from build123d import *

# Parameters (mm, degrees)
SKETCH_R      = 49.5
SKETCH_R_2    = 47
PAD_DEPTH     = 100
SKETCH002_W   = 120
SKETCH002_H   = 120
SKETCH002_R   = 57.5
SKETCH002_R_2 = 2.5
PAD001_DEPTH  = 2.5
FILLET_R      = 4


with BuildPart() as part:
    # Sketch → Pad (new body)
    with BuildSketch(Plane.XY):
        Circle(SKETCH_R)
        Circle(SKETCH_R_2, mode=Mode.SUBTRACT)
    extrude(amount=PAD_DEPTH)

    # Sketch001 → Revolution (revolve)
    with BuildSketch(Plane.XZ):
        with BuildLine():
            ThreePointArc((-57.5, -10.5), (-50.075379, -7.424621), (-47, 0))
            Line((-49.5, 0), (-47, 0))
            ThreePointArc((-57.5, -8), (-51.843146, -5.656854), (-49.5, 0))
            Line((-57.5, -10.5), (-57.5, -8))
        make_face()
    revolve(axis=Axis((0, 0, 0), (0, 0, 1)))

    # Sketch002 (on DatumPlane) → Pad001 (join)
    with BuildSketch(Plane(origin=(0, 0, -10.5), x_dir=(0, -1, 0), z_dir=(0, 0, 1))):
        Rectangle(SKETCH002_W, SKETCH002_H)
        Circle(SKETCH002_R, mode=Mode.SUBTRACT)
        with Locations((-52.499987, 52.500013)):
            Circle(SKETCH002_R_2, mode=Mode.SUBTRACT)
        with Locations((-52.500013, -52.499987)):
            Circle(SKETCH002_R_2, mode=Mode.SUBTRACT)
        with Locations((52.499987, -52.500013)):
            Circle(SKETCH002_R_2, mode=Mode.SUBTRACT)
        with Locations((52.500013, 52.499987)):
            Circle(SKETCH002_R_2, mode=Mode.SUBTRACT)
    extrude(amount=PAD001_DEPTH)

    # Fillet
    fillet_edges = [part.edges().sort_by_distance(p)[0] for p in [
        (-60, -60, -9.25),
        (60, -60, -9.25),
        (-60, 60, -9.25),
        (60, 60, -9.25),
    ]]
    fillet(fillet_edges, radius=FILLET_R)


solid = part.part
Design review of the part built by this model. Coordinates are the model's own, in mm. A direction names the side the tool comes from. Coordinates: 2 decimals unless noted, no trailing zeros. Order: outer loops, then holes, each group sorted by start corner. A loop starts at its lowest first (then second) coordinate and runs counter-clockwise, first axis right, second up.
Item 1: For pin 1 Ø12 at (x, z) = (-25.5, 68) entering from +Y; pin 2 Ø4.5 at (x, y) = (-52.5, -52.5) entering from -Z; pin 3 Ø2 at (x, z) = (-22, 58) entering from +Y; pin 4 Ø8 at (y, z) = (14.5, 67) entering from -X, all flat-tipped, find the tip position at first contact; note any pin that passes through.
Item 2: Take a section at A-A, the plane y = 0. Write out the cut boundary in (x, z), then the cut area to 3 significant figures.
Item 3: For line 1 (X direction, y = 0, z = 75); line 2 (Z direction, x = -31.5, y = 50.5); line 3 (Y direction, x = 39, z = 5.5), list the stretches that pass through material, from the lowest coordinate up.
Item 4: The part is to be moulded in two halves that separate along X. For faces 1 (the cylindrical face through (-58.797, 58.859, -9.232)), 2 (the cylindrical face through (51, 54.5, -9.3)), 3 (the cylindrical face through (-6.44, 49.08, 49.3)), say which applies: pulls with the +X half, pulls with the -X half, needs draft (parallel to the pull), parting line crosses it, or undercut.
Item 5: Take a section at D-D, the plane z = -4. Write out the cut boundary in (x, y), then the cut area to 3 significant figures.
Item 6: Take a section at C-C, the plane z = 14. Write out the cut boundary in (x, y), then the cut area to 3 significant figures.
Item 7: For faces 4 (the flat face through (-22, 54, -8)), 5 (the flat face through (-22, 54, -10.5)), list the 3-axis set-ups (+Z, -Z, +X, -X, +Y, -Y) from which the entire face can be reached by the end or side of a thin tool; tool diameter is ignored.
The answers:
1. pin 1: stops at y = 45.5
1. pin 2: passes through
1. pin 3: stops at y = 44.82
1. pin 4: stops at x = -48.37
2. outline: (-60, -10.5) - (-57.5, -10.5) arc R10.5 ccw to (-47, 0) - (-47, 100) - (-49.5, 100) - (-49.5, 0) arc R8 cw to (-57.5, -8) - (-60, -8) - close; (47, 0) arc R10.5 ccw to (57.5, -10.5) - (60, -10.5) - (60, -8) - (57.5, -8) arc R8 cw to (49.5, 0) - (49.5, 100) - (47, 100) - close
2. area: 585 mm2
3. line 1: x = -49.5 to -47, 47 to 49.5
3. line 2: z = -10.5 to -8
3. line 3: y = -30.48 to -26.23, 26.23 to 30.48
4. face 1: pulls with the -X half
4. face 2: undercut
4. face 3: parting line crosses it
5. outline: circle Ø101.14 at (0, 0); hole circle Ø95.58 at (0, 0)
5. area: 859 mm2
6. outline: circle Ø99 at (0, 0); hole circle Ø94 at (0, 0)
6. area: 758 mm2
7. face 4: +Z
7. face 5: -Z, +X, -X, +Y, -Y
